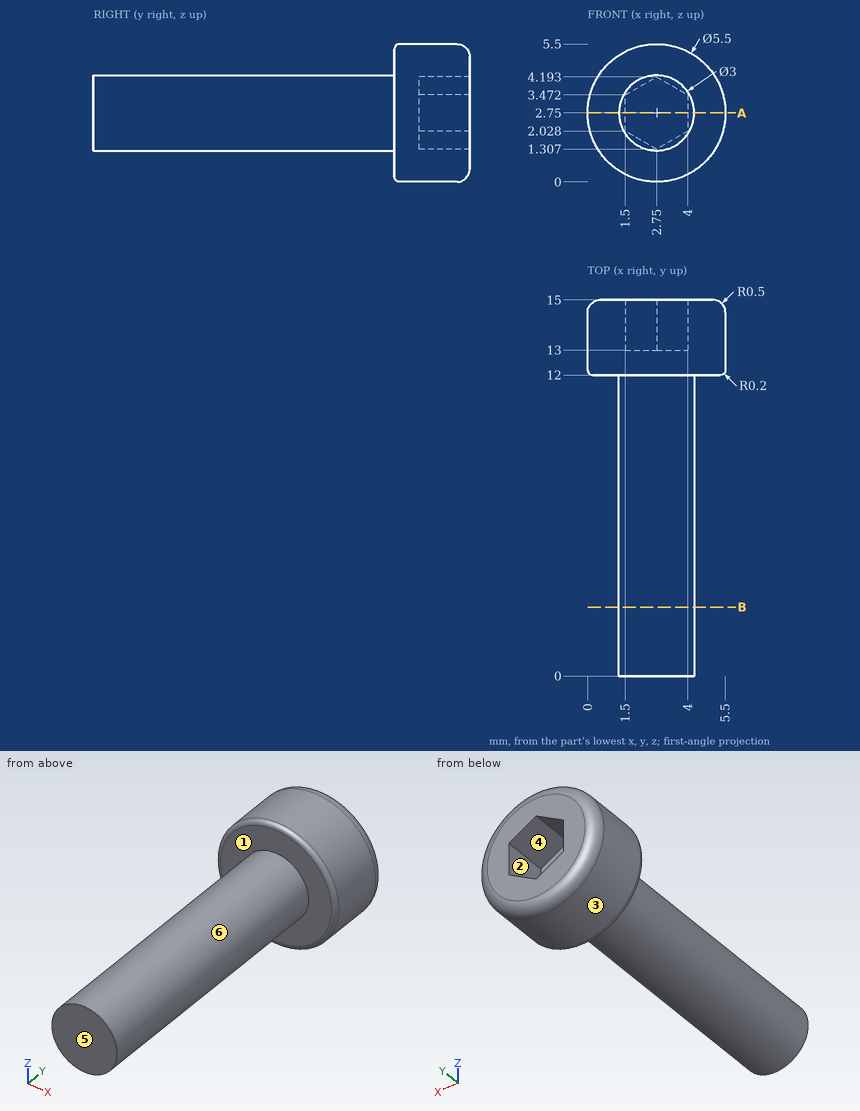
Here's the drawing with two shaded views (mm, measured from the low corner). I have some questions. A direction names the side the tool comes from. Round coordinates to 2 decimals unless told otherwise and drop trailing zeros. Order: outer loops, then holes, each group sorted by start corner. A loop starts at its lowest first (then second) coordinate and runs counter-clockwise, first axis right, second up. Notation, with made-up numbers: (53.5, 84.5) -> (83.5, 84.5) arc R23 cw to (83.5, 109.5) -> close; hole circle Ø10 at (33, 84). An arc over 180 degrees is marked (long way). Write each question's results on one line, items separated by ' | '. Start each with the question number.
Item 1: Which directions (+Z, -Z, +X, -X, +Y, -Y) give clear straight access to the entire face, cutting with the end or side of a thin tool? Please do the marked faces 1, 2 and 3.
Item 2: Will these pins go through, and if not, where does the flat tip stop? pin 1 (1.5 mm diameter, centred on x = 4.5, y = 5.5, fed in from -Z); pin 2 (1.3 mm diameter, centred on x = 3, z = 2.5, fed in from +Y).
Item 3: Thinking about a two-plate mould opening in X: for the marked faces 4, 5 and 6, which applies, +X half, -X half, draft (parallel to the pull), parting line (faces both ways), or undercut?
Item 4: Please list where these lines run through material, in increasing order: L1, parallel to X at y = 13.5, z = 2.9 (1 decimal); L2, parallel to Y at x = 4.1, z = 4; L3, parallel to Y at x = 3.1, z = 1.9.
Item 5: If we section it at A-A, the plane z = 2.75: Write out the boundary of the cut face in (x, y).
Item 6: If we section it at B-B, the plane y = 2.75: Write out the boundary of the cut face in (x, z).
Results:
1) face 1: -Y | face 2: +Y | face 3: +Y, -Y
2) pin 1: stops at z = 1.63 | pin 2: stops at y = 13
3) face 4: undercut | face 5: draft | face 6: parting line
4) L1: x = 0 to 1.5, 4 to 5.5 | L2: y = 12 to 15 | L3: y = 0 to 13
5) outline: (0, 12.2) arc R0.2 ccw to (0.2, 12) -> (1.25, 12) -> (1.25, 0) -> (4.25, 0) -> (4.25, 12) -> (5.3, 12) arc R0.2 ccw to (5.5, 12.2) -> (5.5, 14.5) arc R0.5 ccw to (5, 15) -> (4, 15) -> (4, 13) -> (1.5, 13) -> (1.5, 15) -> (0.5, 15) arc R0.5 ccw to (0, 14.5) -> close
6) outline: circle Ø3 at (2.75, 2.75)
